Source: CAD feature listing. Evaluate the final solid. Frame: model axes, mm. A direction names the side the tool comes from. Give positions to 0.01 mm unless a question says otherwise; leave off trailing zeros. Order: outer loops, then holes, each group sorted by start corner. A loop starts at its lowest first (then second) coordinate and runs counter-clockwise, first axis right, second up. Notation, with made-up numbers: M 65.5,72.5 L 90.5,72.5 A23 ccw 90.5,83.5 Z; hole C 75,-29 d3. An arc over 180 degrees is marked long. Use CSV: the item, a comma, the result in double quotes. Start each with the question number.
Item 1: Section query A-A on x = 0. Return loops of the section in (y, z).
Item 2: Ray query, probe 1 along Y at (x, z) = (0, -5); probe 2 along Y at (x, z) = (-2.5, -3.5); probe 3 along Z at (x, y) = (-3, -7). Return the intervals inside material, ascending. Write a range as from..to.
Item 3: Section query B-B on z = -5.5. Count the separate pieces of the cut face and the enclosed holes in it, and give its area (3 significant figures).
Item 4: First-contact query: pin 1 (7 mm diameter, centred on x = 0, y = 0, fed in from +Z); pin 2 (2 mm diameter, centred on x = 5, z = -5.5, fed in from +Y); pin 3 (3 mm diameter, centred on y = 12.5, z = -5.5, fed in from -X). Flat tips, straight axial feed; report the tip coordinate or a pass-through.
Item 5: Access query for faces 5 (the face through (0, -4, -15)), 6 (the face through (-5.04, 7.52, -6.08)). Directions: +Z, -Z, +X, -X, +Y, -Y. A direction counts if a zero-diameter tool reaches every point of the face in a straight line with its end or side. Return the directions, or none.
Item 6: Pull-direction query (Y, two-part tool) for faces 1 (the face through (-12, -9.2, -0.12)), 2 (the face through (3, -3, 0)), 3 (the face through (-0.867, -3.905, -4.93)), 4 (the face through (11.39, 0.14, -13.37)); classes: +Y half, -Y half, draft (parallel to the pull), parting line (faces both ways), or undercut.
from build123d import *

# Parameters (mm, degrees)
F0_R           = 17.5
F1_DEPTH       = 15
F2_D           = 5.5
F2_DEPTH       = 12
F2_TIP         = 1.6523667023
F3_D           = 7
F3_DEPTH       = 12
F3_TIP         = 2.1030121666
F4_D           = 4
F4_DEPTH       = 12
F4_TIP         = 1.2017212381
F5_D           = 3.5
F5_CBORE_D     = 8
F5_CBORE_DEPTH = 10
F6_SIZE        = 2.5


with BuildPart() as f1:
    # F0 (on Top) → F1 (new body)
    with BuildSketch(Plane.XY):
        Circle(F0_R)
    extrude(amount=-F1_DEPTH)

    # F2
    with Locations(Plane.XY):
        with Locations((10.9375, 0)):
            Hole(F2_D / 2, depth=F2_DEPTH)
            with Locations((0, 0, -(F2_DEPTH + F2_TIP / 2))):  # 118° drill point
                Cone(0, F2_D / 2, F2_TIP, mode=Mode.SUBTRACT)

    # F3
    with Locations(Plane.XY):
        with Locations((-4.375, -7.5777222831)):
            Hole(F3_D / 2, depth=F3_DEPTH)
            with Locations((0, 0, -(F3_DEPTH + F3_TIP / 2))):  # 118° drill point
                Cone(0, F3_D / 2, F3_TIP, mode=Mode.SUBTRACT)

    # F4
    with Locations(Plane.XY):
        with Locations((-5.46875, 9.4721528539)):
            Hole(F4_D / 2, depth=F4_DEPTH)
            with Locations((0, 0, -(F4_DEPTH + F4_TIP / 2))):  # 118° drill point
                Cone(0, F4_D / 2, F4_TIP, mode=Mode.SUBTRACT)

    # F5 (through all)
    with Locations(Plane.XY):
        with Locations((0, 0)):
            CounterBoreHole(F5_D / 2, F5_CBORE_D / 2, F5_CBORE_DEPTH)

    # F6
    f6_edges = [f1.edges().sort_by_distance(p)[0] for p in [
        (-17.5, 0, 0),
    ]]
    chamfer(f6_edges, length=F6_SIZE)


solid = f1.part
Verdict:
1,outline,"M -17.5,-15 L -1.75,-15 L -1.75,-10 L -4,-10 L -4,0 L -15,0 L -17.5,-2.5 Z; M 1.75,-15 L 17.5,-15 L 17.5,-2.5 L 15,0 L 4,0 L 4,-10 L 1.75,-10 Z"
2,probe 1,"-17.5..-4, 4..17.5"
2,probe 2,"-17.32..-10.53, -4.62..-3.12, 3.12..17.32"
2,probe 3,"-15..-13.21"
3,separate pieces,"1"
3,enclosed holes,"4"
3,area,"837 mm2"
4,pin 1,"z = -10"
4,pin 2,"y = 17.04"
4,pin 3,"x = -13.61"
5,face 5,"-Z, +X, -X, +Y, -Y"
5,face 6,"+Z"
6,face 1,"parting line"
6,face 2,"draft"
6,face 3,"undercut"
6,face 4,"undercut"
